Geometry check sheet. Reference: drawing and pictorial views, mm from the part's lowest x, y, z. Give positions to 0.01 mm unless a question says otherwise; leave off trailing zeros. Write each loop counter-clockwise with the first axis right and the second up, starting at its lowest first coordinate (ties: lowest second). Pieces come first, ordered by that corner, then holes. Notation, with made-up numbers: (-17.75, 73.5) - (-12.75, 73.5) arc R29 cw to (-12.75, 97.5) - close; hole circle Ø6 at (86.5, 28). An arc over 180 degrees is marked (long way). Put each result on its own line as item: value.
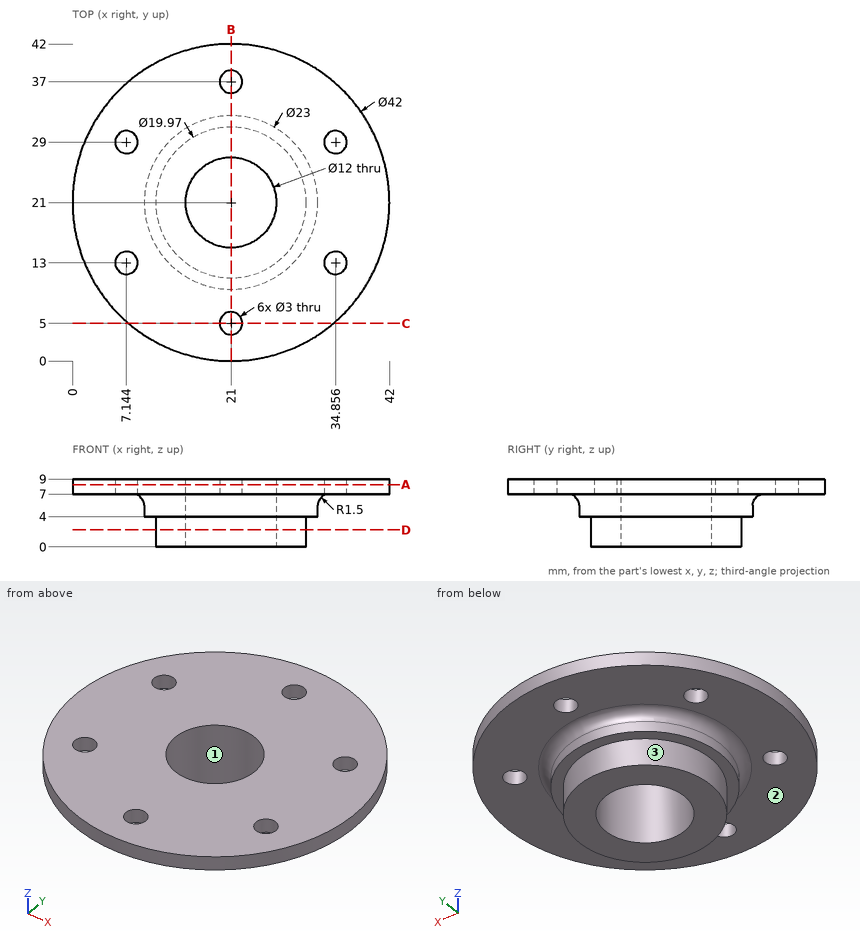
Q1. Go/stop test with a flat-tipped pin: pin 1 Ø4 at (x, y) = (7.14, 29) entering from -Z. Record where the tip stops, or that it passes through.
Answers follow:
pin 1: stops at z = 7
Q2. Section check D-D, the plane z = 2.25. Record the cut outline in (x, y) (1 decimal).
Answers follow:
outline: circle Ø20 at (21, 21); hole circle Ø12 at (21, 21)
Q3. Section check A-A, the plane z = 8.25. Record the cut outline in (x, y), plus the area to 3 significant figures.
Answers follow:
outline: circle Ø42 at (21, 21); hole circle Ø3 at (7.14, 13); hole circle Ø3 at (7.14, 29); hole circle Ø12 at (21, 21); hole circle Ø3 at (21, 5); hole circle Ø3 at (21, 37); hole circle Ø3 at (34.86, 13); hole circle Ø3 at (34.86, 29)
area: 1,230 mm2
Q4. Release check for a two-part mould opening along X. For the marked faces 1, 2 and 3 record: released by +X, released by -X, zero draft, split by the parting line, or undercut.
Answers follow:
face 1: undercut
face 2: zero draft
face 3: split by the parting line
Q5. Section check B-B, the plane x = 21. Record the cut outline in (y, z) (1 decimal).
Answers follow:
outline: (0, 7) - (3.5, 7) - (3.5, 9) - (0, 9) - close; (6.5, 7) - (8, 7) arc R1.5 cw to (9.5, 5.5) - (9.5, 4) - (11, 4) - (11, 0) - (15, 0) - (15, 9) - (6.5, 9) - close; (27, 0) - (31, 0) - (31, 4) - (32.5, 4) - (32.5, 5.5) arc R1.5 cw to (34, 7) - (35.5, 7) - (35.5, 9) - (27, 9) - close; (38.5, 7) - (42, 7) - (42, 9) - (38.5, 9) - close
Q6. Section check C-C, the plane y = 5. Record the cut outline in (x, z).
Answers follow:
outline: (7.4, 7) - (19.5, 7) - (19.5, 9) - (7.4, 9) - close; (22.5, 7) - (34.6, 7) - (34.6, 9) - (22.5, 9) - close
Q7. Scan lines: line 1 along Y through (x, z) = (21, 7.9); line 2 along Y through (x, z) = (21, 4.25); line 3 along Z through (x, y) = (7.5, 25.5). Record each from-to range of solid material in increasing order.
Answers follow:
line 1: y = 0 to 3.5, 6.5 to 15, 27 to 35.5, 38.5 to 42
line 2: y = 9.5 to 15, 27 to 32.5
line 3: z = 7 to 9
